Work out the finished part from the listing and answer in its coordinate system (mm). A direction names the side the tool comes from. Coordinates: 2 decimals unless noted, no trailing zeros. Order: outer loops, then holes, each group sorted by start corner. A loop starts at its lowest first (then second) coordinate and runs counter-clockwise, first axis right, second up. Notation, with made-up numbers: (38, 41.5) -> (50, 41.5) arc R31 cw to (50, 70.5) -> close; hole circle Ø11 at (29, 16). An arc over 180 degrees is marked (long way). Answer as CSV lines item,"result". Start each with the question number.
Item 1: Straight lines are drawn through the part: L1, parallel to X at y = 11.75, z = 0; L2, parallel to Y at x = 6.25, z = 0.5; L3, parallel to X at y = 9.5, z = 1.5. For each, find the intervals that lie inside material, in ascending order.
Item 2: Section D-D (x = 9.5) is taken. Write down the section's boundary in (y, z).
Item 3: Which of the six approach directions +Z, -Z, +X, -X, +Y, -Y give full straight-line access (tool end or side, diameter ignored) to faces 1 (the face through (2, 0, -2)), 2 (the face through (6, -1, -5))?
Item 4: For a pull along X with two mould halves and no side action, classify faces 3 (the face through (10.083, -1.479, -2.535)), 4 (the face through (3.926, 7.888, 0.766)), 5 (the face through (6, -1, 5)) as pulls with the +X half, pulls with the -X half, needs draft (parallel to the pull), parting line crosses it, or undercut.
Item 5: Section A-A (y = 10.75) is taken. Write down the section's boundary in (x, z), then the cut area to 3 significant figures.
Item 6: Section B-B (z = 3) is taken. Write down the section's boundary in (x, y), then the cut area to 3 significant figures.
Item 7: Each of these flat-tipped pins is pushed along its axis until it touches: pin 1 Ø4 at (x, y) = (9, 4) entering from -Z; pin 2 Ø4 at (y, z) = (2.5, 2) entering from +X. Where does it stop, or does it pass through?
Item 8: Section C-C (y = -0.5) is taken. Write down the section's boundary in (x, z).
Autodesk Inventor part; units mm, degrees
ref_plane "YZ Plane" through (0, 0, 0) normal (1, 0, 0) x (0, 1, 0)
ref_plane "XZ Plane" through (0, 0, 0) normal (0, 1, 0) x (-1, 0, 0)
ref_plane "XY Plane" through (0, 0, 0) normal (0, 0, 1) x (1, 0, 0)
sketch "Sketch1" plane through (0, 0, 0) normal (0, 1, 0) x (-1, 0, 0)
  line L0 (0, 0) -> (-11.547, 0)
  line L1 (-11.547, 0) -> (-8.6603, 5)
  line L2 (-8.6603, 5) -> (-2.8868, 5)
  line L3 (-2.8868, 5) -> (0, 0)
  line L4 (0, 0) -> (-2.8868, -5)
  line L5 (-2.8868, -5) -> (-8.6603, -5)
  line L6 (-8.6603, -5) -> (-11.547, 0)
  circle A0 centre (-5.7735, 0) radius 4
  circle A1 centre (-5.7735, 0) radius 2
  dimension "d0" = 10
  dimension "d1" = 8
  dimension "d2" = 4
extrude "Extrusion1" add sketch "Sketch1" against normal blind 3
extrude "Extrusion2" add sketch "Sketch1" along normal blind 16 contours A0 L0 A1 | L0 A1 A0
thread "Thread1"
properties part number "HUDSON-1-87"
Checked values:
1,L1,"x = 1.77 to 3.77, 7.77 to 9.77"
1,L2,"y = -3 to 0"
1,L3,"x = 2.07 to 4.45, 7.1 to 9.48"
2,outline,"(-3, -3.55) -> (0, -3.55) -> (0, -1.45) -> (16, -1.45) -> (16, 1.45) -> (0, 1.45) -> (0, 3.55) -> (-3, 3.55) -> close"
3,face 1,"+Y"
3,face 2,"-Z, +X, -X, +Y, -Y"
4,face 3,"pulls with the +X half"
4,face 4,"undercut"
4,face 5,"needs draft"
5,outline,"circle Ø8 at (5.77, 0); hole circle Ø4 at (5.77, 0)"
5,area,"37.7 mm^2"
6,outline,"(1.73, -3) -> (9.81, -3) -> (9.81, 0) -> (8.42, 0) -> (8.42, 16) -> (3.13, 16) -> (3.13, 0) -> (1.73, 0) -> close"
6,area,"109 mm^2"
7,pin 1,"stops at z = -3.81"
7,pin 2,"stops at x = 9.77"
8,outline,"(0, 0) -> (2.89, -5) -> (8.66, -5) -> (11.55, 0) -> (8.66, 5) -> (2.89, 5) -> close"
